Geometry check sheet. Reference: the model listing, model coordinates, mm. Face numbers are marked on the shaded views. A direction names the side the tool comes from. Round coordinates to 2 decimals unless told otherwise and drop trailing zeros. Order: outer loops, then holes, each group sorted by start corner. A loop starts at its lowest first (then second) coordinate and runs counter-clockwise, first axis right, second up. Notation, with made-up numbers: (49, -39) - (78, -39) arc R26 cw to (78, 0) - close; hole circle Ø8 at (1.5, 69.5). An arc over 180 degrees is marked (long way). Return JSON: item names as keys, results as strings. Group by question number.
Q1. Sectioned sample at B-B, the plane y = 14. Record the cut outline in (x, z), then the cut area to 3 significant figures.
Q2. Material ranges on line 1 along Y through (x, z) = (-4.5, 10.75); line 2 along Z through (x, y) = (-4, 5.5); line 3 along Y through (x, z) = (0, 14.5), recorded low to high.
Q3. Tool access check on the marked faces 1, 2, 3, 4 and 5. Record the directions out of +Z, -Z, +X, -X, +Y, -Y that give a thin tool (end or side, any length) a straight path to the whole face; none if there is none.
Q4. Gauge pin test, flat ends, axial feed: pin 1 Ø5 at (x, y) = (-5, -6) entering from +Z; pin 2 Ø0.6 at (y, z) = (12, 1.5) entering from +X; pin 3 Ø4 at (x, z) = (2.5, 9.5) entering from +Y. Record the tip position at first contact, or that the pin passes through.
Q5. Sectioned sample at A-A, the plane x = 0. Give the number of separate pieces and of enclosed holes in the cut face, then the cut area to 3 significant figures.
Q6. Sectioned sample at C-C, the plane z = 4. Record the cut outline in (x, y), then the cut area to 3 significant figures.
Q7. Draft check along X on the marked faces 6, 7, 8 and 9. Enter one of: pulls with the +X half, pulls with the -X half, needs draft (parallel to the pull), parting line crosses it, or undercut.
Q8. Sectioned sample at D-D, the plane x = 6.75. Record the cut outline in (y, z), then the cut area to 3 significant figures.
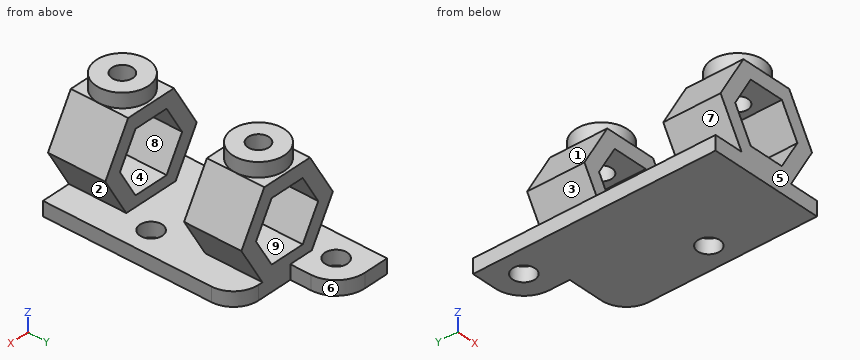
```python
from build123d import *

# Parameters (mm, degrees)
SKETCH1_W           = 16
SKETCH1_H           = 33.8605711
SKETCH1_R           = 1.55
BOSS_EXTRUDE1_DEPTH = 2
BOSS_EXTRUDE2_DEPTH = 8
BOSS_EXTRUDE3_START = 11
BOSS_EXTRUDE3_DEPTH = 8
CUT_EXTRUDE1_REACH  = 25.38
SKETCH4_R           = 1.45
CUT_EXTRUDE2_REACH  = 24.24
FILLET1_R           = 3.5
BOSS_EXTRUDE4_START = 2
SKETCH6_R           = 3.608439182
SKETCH6_R_2         = 1.45
BOSS_EXTRUDE4_DEPTH = 2


with BuildPart() as part:
    # Sketch1 → Boss-Extrude1 (new body)
    with BuildSketch(Plane.XY):
        Rectangle(SKETCH1_W, SKETCH1_H)
        with Locations((-4.5, 12.93028555)):
            Circle(SKETCH1_R, mode=Mode.SUBTRACT)
        with Locations((4.5, -4.93028555)):
            Circle(SKETCH1_R, mode=Mode.SUBTRACT)
    extrude(amount=BOSS_EXTRUDE1_DEPTH)

    # Sketch2 → Boss-Extrude2 (add)
    with BuildSketch(Plane.XZ.offset(16.93028555)):
        Polygon((-3.608439182, 14), (-7.216878365, 7.75), (-3.897114317, 2), (3.897114317, 2), (7.216878365, 7.75), (3.608439182, 14), align=None)
        Polygon((-2.453738644, 3.5), (2.453738644, 3.5), (4.907477288, 7.75), (2.453738644, 12), (-2.453738644, 12), (-4.907477288, 7.75), align=None, mode=Mode.SUBTRACT)
    extrude(amount=-BOSS_EXTRUDE2_DEPTH)

    # Sketch3 → Boss-Extrude3 (add)
    with BuildSketch(Plane(origin=(0, -8.93028555, 0), x_dir=(1, 0, 0), z_dir=(0, 1, 0)).offset(BOSS_EXTRUDE3_START)):
        Polygon((-3.608439182, -14), (3.608439182, -14), (7.216878365, -7.75), (3.897114317, -2), (-3.897114317, -2), (-7.216878365, -7.75), align=None)
        Polygon((-4.907477288, -7.75), (-2.453738644, -12), (2.453738644, -12), (4.907477288, -7.75), (2.453738644, -3.5), (-2.453738644, -3.5), align=None, mode=Mode.SUBTRACT)
    extrude(amount=BOSS_EXTRUDE3_DEPTH)

    # Sketch4 → Cut-Extrude1 (cut, up to next)
    with BuildSketch(Plane.XY.offset(14), mode=Mode.PRIVATE) as cut_extrude1_sk1:
        with Locations((0, -12.93028555)):
            Circle(SKETCH4_R)
    cut_extrude1_tool1 = extrude(cut_extrude1_sk1.sketch, amount=-CUT_EXTRUDE1_REACH, mode=Mode.PRIVATE) & part.part
    # Sketch4 → Cut-Extrude1 (cut, up to next)
    with BuildSketch(Plane.XY.offset(14), mode=Mode.PRIVATE) as cut_extrude1_sk2:
        with Locations((0, 6.06971445)):
            Circle(SKETCH4_R)
    cut_extrude1_tool2 = extrude(cut_extrude1_sk2.sketch, amount=-CUT_EXTRUDE1_REACH, mode=Mode.PRIVATE) & part.part
    add(cut_extrude1_tool1.solids().sort_by_distance((0, -12.930286, 14))[0], mode=Mode.SUBTRACT)
    add(cut_extrude1_tool2.solids().sort_by_distance((0, 6.069714, 14))[0], mode=Mode.SUBTRACT)

    # Sketch5 → Cut-Extrude2 (cut, up to next)
    with BuildSketch(Plane.XY.offset(2), mode=Mode.PRIVATE) as cut_extrude2_sk1:
        with BuildLine():
            Line((-0.5, 12.93028555), (-0.5, 10.06971445))
            Line((-0.5, 10.06971445), (8, 10.06971445))
            Line((8, 10.06971445), (8, 16.93028555))
            Line((8, 16.93028555), (-4.5, 16.93028555))
            ThreePointArc((-4.5, 16.93028555), (-1.671572875, 15.758712674), (-0.5, 12.93028555))
        make_face()
    cut_extrude2_tool1 = extrude(cut_extrude2_sk1.sketch, amount=-CUT_EXTRUDE2_REACH, mode=Mode.PRIVATE) & part.part
    add(cut_extrude2_tool1.solids().sort_by_distance((3.463989, 13.641064, 2))[0], mode=Mode.SUBTRACT)

    # Fillet1
    fillet1_edges = [part.edges().sort_by_distance(p)[0] for p in [
        (8, 10.06971445, 1),
    ]]
    fillet(fillet1_edges, radius=FILLET1_R)

    # Sketch6 → Boss-Extrude4 (add)
    # profile 1 of 2: a face of its own
    with BuildSketch(Plane.XY.offset(14).offset(BOSS_EXTRUDE4_START)):
        with Locations((0, 6.06971445)):
            Circle(SKETCH6_R)
        with Locations((0, 6.06971445)):
            Circle(SKETCH6_R_2, mode=Mode.SUBTRACT)
    # profile 2 of 2: a face of its own
    with BuildSketch(Plane.XY.offset(14).offset(BOSS_EXTRUDE4_START)):
        with Locations((0, -12.93028555)):
            Circle(SKETCH6_R)
        with Locations((0, -12.93028555)):
            Circle(SKETCH6_R_2, mode=Mode.SUBTRACT)
    extrude(amount=-BOSS_EXTRUDE4_DEPTH)


solid = part.part
```
Reply:
{
 "1": {"outline": "(-8, 0) - (-5.62, 0) - (-5.62, 2) - (-8, 2) - close; (-3.38, 0) - (-0.65, 0) - (-0.65, 2) - (-3.38, 2) - close", "area": "10.2 mm^2"},
 "2": {"line 1": "-16.93 to -8.93, 2.07 to 10.07", "line 2": "0 to 2, 2.18 to 6.18, 9.32 to 13.32", "line 3": "-16.54 to -14.38, -11.48 to -9.32, 2.46 to 4.62, 7.52 to 9.68"},
 "3": {"face 1": "+Z, -X, +Y, -Y", "face 2": "+X, +Y, -Y", "face 3": "-X, +Y, -Y", "face 4": "+Y, -Y", "face 5": "+Z, -Z, +X, -X, -Y"},
 "4": {"pin 1": "z = 2", "pin 2": "x = -0.5", "pin 3": "y = 10.07"},
 "5": {"separate pieces": "5", "enclosed holes": "0", "area": "116 mm^2"},
 "6": {"outline": "(-5.05, -16.93) - (-2.74, -16.93) - (-2.74, -8.93) - (-5.05, -8.93) - close; (-5.05, 2.07) - (-2.74, 2.07) - (-2.74, 10.07) - (-5.05, 10.07) - close; (2.74, -16.93) - (5.05, -16.93) - (5.05, -8.93) - (2.74, -8.93) - close; (2.74, 2.07) - (5.05, 2.07) - (5.05, 10.07) - (2.74, 10.07) - close", "area": "73.9 mm^2"},
 "7": {"face 6": "pulls with the +X half", "face 7": "pulls with the -X half", "face 8": "undercut", "face 9": "undercut"},
 "8": {"outline": "(-16.93, 0) - (9.25, 0) - (9.25, 2) - (-16.93, 2) - close; (-16.93, 6.94) - (-8.93, 6.94) - (-8.93, 8.56) - (-16.93, 8.56) - close; (2.07, 6.94) - (10.07, 6.94) - (10.07, 8.56) - (2.07, 8.56) - close", "area": "78.2 mm^2"}
}
